from build123d import *

# Parameters (mm, degrees)
BOSS_EXTRUDE1_DEPTH = 15
CUT_EXTRUDE1_DEPTH  = 10
SKETCH3_R           = 1
CUT_EXTRUDE2_DEPTH  = 10


with BuildPart() as part:
    # Sketch1 → Boss-Extrude1 (new body)
    with BuildSketch(Plane(origin=(0, 0, 0), x_dir=(1, 0, 0), z_dir=(0, 1, 0))):
        with BuildLine():
            ThreePointArc((-35.496119508, 46.04177293), (0, 20.636213797), (35.496119508, 46.04177293))
            ThreePointArc((35.496119508, 46.04177293), (0, -58.136213797), (-35.496119508, 46.04177293))
        make_face()
    extrude(amount=BOSS_EXTRUDE1_DEPTH)

    # Sketch2 → Cut-Extrude1 (cut)
    with BuildSketch(Plane.XZ):
        with BuildLine():
            Line((7.448979486, 1), (4.898979486, 1))
            ThreePointArc((4.898979486, 1), (-5, 0), (4.898979486, -1))
            Line((4.898979486, -1), (7.448979486, -1))
            Line((7.448979486, -1), (7.448979486, 1))
        make_face()
    extrude(amount=-CUT_EXTRUDE1_DEPTH, mode=Mode.SUBTRACT)

    # Sketch3 → Cut-Extrude2 (cut)
    with BuildSketch(Plane(origin=(0, 15, 0), x_dir=(1, 0, 0), z_dir=(0, 1, 0))):
        with Locations(Location((0, 0, 0), (0, 0, 270))):
            Circle(SKETCH3_R)
    extrude(amount=-CUT_EXTRUDE2_DEPTH, mode=Mode.SUBTRACT)


solid = part.part
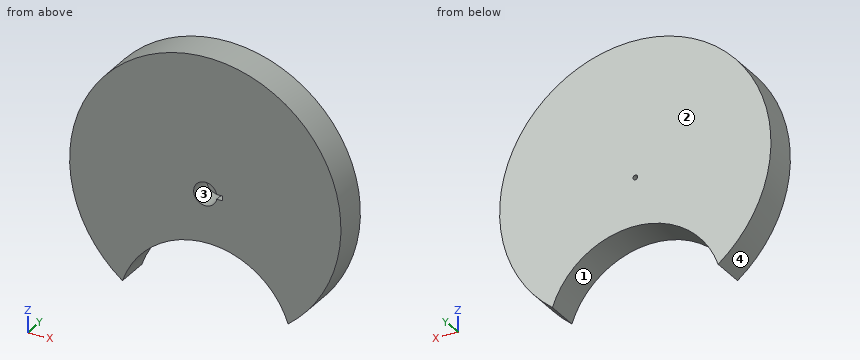
Could you check a few things on this model? Use its own coordinates, in mm. Face numbers are marked on the shaded views. Give positions to 0.01 mm unless a question says otherwise; leave off trailing zeros. Write each loop counter-clockwise with the first axis right and the second up, starting at its lowest first coordinate (ties: lowest second). Pieces come first, ordered by that corner, then holes. Notation, with made-up numbers: (-35.5, 35.5) - (-0.5, 35.5) arc R27 cw to (-0.5, 57.5) - close; hole circle Ø3 at (86.25, 71). An arc over 180 degrees is marked (long way). Use CSV: the item, a comma, the result in double quotes. Start each with the question number.
Item 1: I'm going to push flat-ended pins straight in: pin 1 (1.5 mm diameter, centred on x = 31.5, y = 13.5, fed in from -Z); pin 2 (1.5 mm diameter, centred on x = -15.5, y = 10, fed in from -Z); pin 3 (6 mm diameter, centred on y = 10, z = -21, fed in from +X). Where does each tip first touch, or does it pass through?
Item 2: If I drill on line 1 along X through (y, z) = (5, 0); line 2 along X through (y, z) = (12.45, 0); line 3 along X through (y, z) = (9, 28.5), over which ranges is the centre line in solid material (lowest first)?
Item 3: I want a section at D-D, the plane z = 49. Please give me the cut outline in (x, y).
Item 4: I want a section at C-C, the plane x = -41. Please give me the cut outline in (y, z).
Item 5: If we mould it in two halves opening along Z, with no side actions, what happens to the marked faces 1, 2, 3 and 4? For each: pulls with the +Z half, pulls with the -Z half, needs draft (parallel to the pull), parting line crosses it, or undercut.
Item 6: I want a section at A-A, the plane y = 8. Please give me the cut outline in (x, z).
Item 7: I want a section at B-B, the plane z = -27. Please give me the cut outline in (x, y).
Findings:
1,pin 1,"stops at z = -39"
1,pin 2,"stops at z = -24.34"
1,pin 3,"stops at x = 55.28"
2,line 1,"x = -58.14 to -5, 7.45 to 58.14"
2,line 2,"x = -58.14 to -1, 1 to 58.14"
2,line 3,"x = -50.67 to 50.67"
3,outline,"(-31.29, 0) - (31.29, 0) - (31.29, 15) - (-31.29, 15) - close"
4,outline,"(0, -41.22) - (15, -41.22) - (15, 41.22) - (0, 41.22) - close"
5,face 1,"pulls with the -Z half"
5,face 2,"needs draft"
5,face 3,"undercut"
5,face 4,"parting line crosses it"
6,outline,"(-35.5, -46.04) arc R37.5 cw to (35.5, -46.04) arc R58.14 ccw (long way) to start; hole (4.9, -1) - (7.45, -1) - (7.45, 1) - (4.9, 1) arc R5 ccw (long way) to start"
7,outline,"(-51.49, 0) - (-20.9, 0) - (-20.9, 15) - (-51.49, 15) - close; (20.9, 0) - (51.49, 0) - (51.49, 15) - (20.9, 15) - close"
